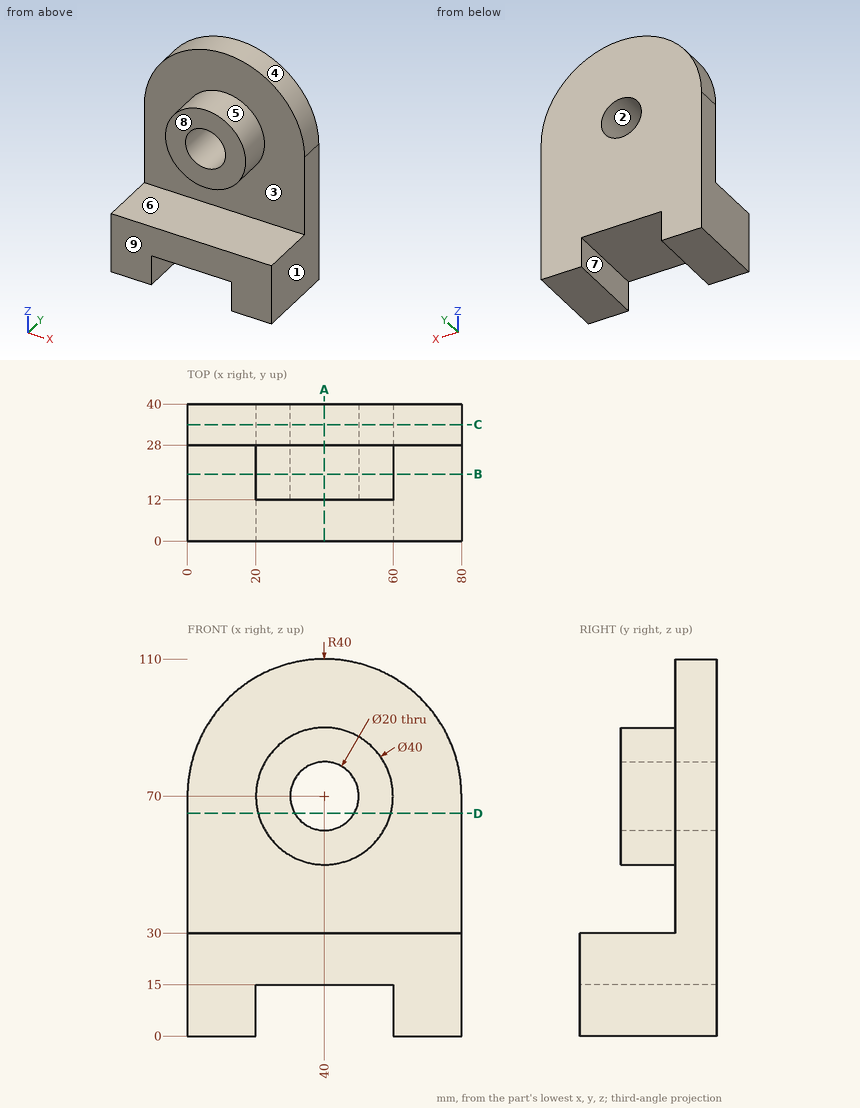
Could you check a few things on this drawing? It's one solid part, dimensions in mm from its lowest x, y, z. A direction names the side the tool comes from. Round coordinates to 2 decimals unless told otherwise and drop trailing zeros. Write each loop counter-clockwise with the first axis right and the second up, starting at its lowest first coordinate (ties: lowest second). Pieces come first, ordered by that corner, then holes. Notation, with made-up numbers: (74.25, -6) -> (128.25, -6) arc R17 cw to (128.25, 6) -> close; hole circle Ø5 at (-24.5, 52). An arc over 180 degrees is marked (long way). One line per question, with ' | ' between items. Start each with the question number.
1) Suppose I cut it at C-C on y = 34. Write out the boundary of the cut face in (x, z).
2) I'm going to push flat-ended pins straight in: P1, Ø8, axis at y = 35.5, z = 75, coming from the -X side; P2, Ø12, axis at x = 47.5, y = 27, coming from the -Z side; P3, Ø4, axis at x = 45, y = 24, coming from the +Z side. Where does each tip first touch, or does it pass through?
3) Suppose I cut it at D-D on z = 65. Write out the boundary of the cut face in (x, y).
4) Suppose I cut it at A-A on x = 40. Write out the boundary of the cut face in (y, z), then the cut area to 3 significant figures.
5) On a 3-axis mill with a long thin cutter (end or side, diameter ignored), from which of +Z, -Z, +X, -X, +Y, -Y can I reach the whole of each face in a straight line? I mean the marked faces 5, 6, 7, 8 and 9. Say none if no direction works.
6) If we mould it in two halves opening along X, with no side actions, what happens to the marked faces 1, 2, 3 and 4? For each: released by +X, released by -X, zero draft, split by the parting line, or undercut.
7) Suppose I cut it at B-B on y = 19.5. Write out the boundary of the cut face in (x, z), then the cut area to 3 significant figures.
8) I need wall thicknesses on line 1 (X direction, y = 5, z = 13.5); line 2 (Y direction, x = 20, z = 100.5); line 3 (Z direction, x = 8, y = 13.5). Which ranges of each line are inside material? Lowest first, please. Write a range as [from, to].
Return value:
1) outline: (0, 0) -> (20, 0) -> (20, 15) -> (60, 15) -> (60, 0) -> (80, 0) -> (80, 70) arc R40 ccw to (0, 70) -> close; hole circle Ø20 at (40, 70)
2) P1: stops at x = 0.01 | P2: stops at z = 15 | P3: stops at z = 89.77
3) outline: (0, 28) -> (20.64, 28) -> (20.64, 12) -> (31.34, 12) -> (31.34, 40) -> (0, 40) -> close; (48.66, 12) -> (59.36, 12) -> (59.36, 28) -> (80, 28) -> (80, 40) -> (48.66, 40) -> close
4) outline: (0, 15) -> (40, 15) -> (40, 60) -> (12, 60) -> (12, 50) -> (28, 50) -> (28, 30) -> (0, 30) -> close; (12, 80) -> (40, 80) -> (40, 110) -> (28, 110) -> (28, 90) -> (12, 90) -> close | area: 1,640 mm2
5) face 5: -Y | face 6: +X, -X, -Y | face 7: -Z, +Y, -Y | face 8: +Z, +X, -X, -Y | face 9: +Z, -Z, +X, -X, -Y
6) face 1: released by +X | face 2: undercut | face 3: zero draft | face 4: split by the parting line
7) outline: (0, 0) -> (20, 0) -> (20, 15) -> (60, 15) -> (60, 0) -> (80, 0) -> (80, 30) -> (0, 30) -> close; circle Ø40 at (40, 70); hole circle Ø20 at (40, 70) | area: 2,740 mm2
8) line 1: x = [0, 20], [60, 80] | line 2: y = [28, 40] | line 3: z = [0, 30]
